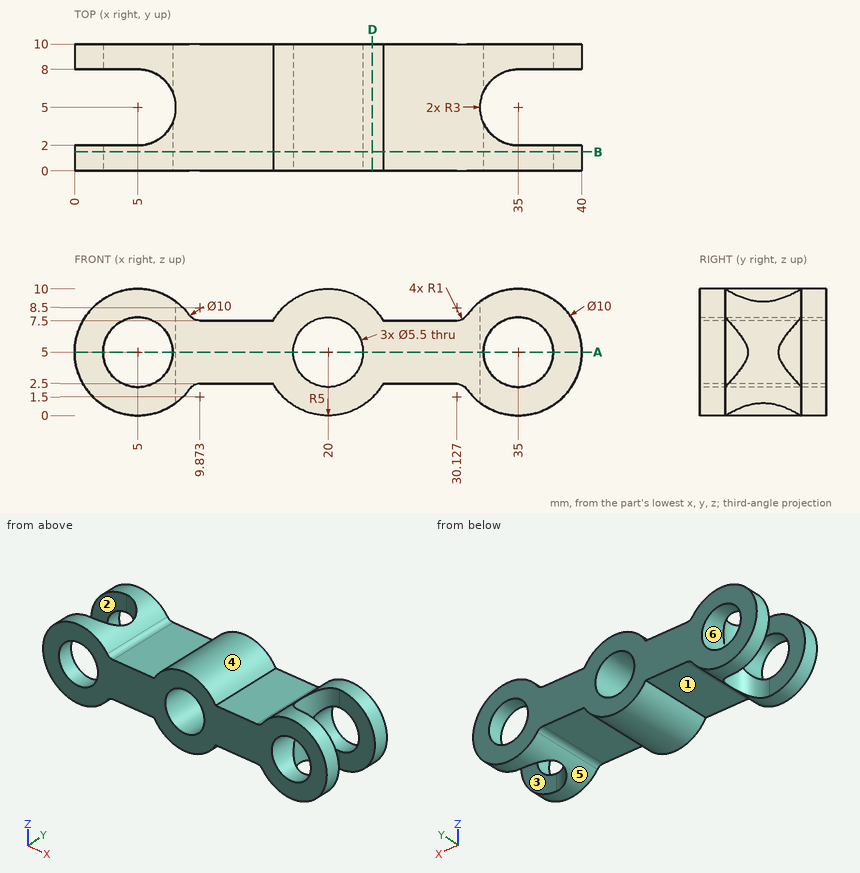
Job drawing, mm, ordinate dimensions from the low corner. One solid piece. A direction names the side the tool comes from. Round coordinates to 2 decimals unless told otherwise and drop trailing zeros. Loops run counter-clockwise (first coordinate to the right, second up) from the corner with the lowest first, then second, coordinate; pieces in that order, holes last.
(1) Which spindle directions (+Z, -Z, +X, -X, +Y, -Y) get a long thin tool onto all of the face, cutting with end or side? Do the marked faces 1, 2 and 3. Say none if no direction does.
(2) Drop flat-ended pins along their axis: pin 1 (3.5 mm diameter, centred on x = 5, z = 5, fed in from +Y); pin 2 (4 mm diameter, centred on y = 5.5, z = 4, fed in from -X); pin 3 (3 mm diameter, centred on x = 28.5, y = 6, fed in from -Z); pin 4 (5 mm diameter, centred on y = 6.5, z = 8, fed in from +X). Give the stop position or say it passes through.
(3) Cut at A-A (z = 5). Give the cut face in (x, y), plus the area to 3 significant figures.
(4) Cut at D-D (x = 23.5). Give the cut face in (y, z).
(5) Wall check: line 1 along X through (y, z) = (6.5, 5); line 2 along X through (y, z) = (7.5, 9); line 3 along X through (y, z) = (7, 1.25) (1 decimal). Give the ranges that are in metal, low to high.
(6) Cut at B-B (y = 1.5). Give the cut face in (x, z), plus the area to 3 significant figures.
(7) Two-plate mould, pull along Z, no slides. Class the marked faces 4, 5 and 6: +Z half, -Z half, draft (parallel to the pull), parting line (faces both ways), or undercut.
Findings below:
1. face 1: -Z, +Y, -Y
1. face 2: +Z, -Z, -X
1. face 3: +Z, -Z, +X
2. pin 1: passes through
2. pin 2: stops at x = 6.96
2. pin 3: stops at z = 2.5
2. pin 4: stops at x = 39.9
3. outline: (0, 0) - (2.25, 0) - (2.25, 2) - (0, 2) - close; (0, 8) - (2.25, 8) - (2.25, 10) - (0, 10) - close; (7.75, 0) - (17.25, 0) - (17.25, 10) - (7.75, 10) - (7.75, 6.2) arc R3 cw to (7.75, 3.8) - close; (22.75, 0) - (32.25, 0) - (32.25, 3.8) arc R3 cw to (32.25, 6.2) - (32.25, 10) - (22.75, 10) - close; (37.75, 0) - (40, 0) - (40, 2) - (37.75, 2) - close; (37.75, 8) - (40, 8) - (40, 10) - (37.75, 10) - close
3. area: 207 mm2
4. outline: (0, 1.43) - (10, 1.43) - (10, 8.57) - (0, 8.57) - close
5. line 1: x = 7.75 to 17.25, 22.75 to 32.25
5. line 2: x = 6.66 to 8, 17 to 23, 32 to 33.34
5. line 3: x = 7.2 to 8.3, 16.7 to 23.3, 31.7 to 32.8
6. outline: (9.06, 2.08) arc R1 cw to (9.87, 2.5) - (15.67, 2.5) arc R5 ccw to (24.33, 2.5) - (30.13, 2.5) arc R1 cw to (30.94, 2.08) arc R5 ccw (long way) to (30.94, 7.92) arc R1 cw to (30.13, 7.5) - (24.33, 7.5) arc R5 ccw to (15.67, 7.5) - (9.87, 7.5) arc R1 cw to (9.06, 7.92) arc R5 ccw (long way) to start; hole circle Ø5.5 at (5, 5); hole circle Ø5.5 at (20, 5); hole circle Ø5.5 at (35, 5)
6. area: 219 mm2
7. face 4: +Z half
7. face 5: parting line
7. face 6: undercut
